Check sheet for the drawn part. Datum: minimum x, y, z corner. Units: mm. A direction names the side the tool comes from. Give positions to 0.01 mm unless a question says otherwise; leave off trailing zeros. Write each loop counter-clockwise with the first axis right and the second up, starting at its lowest first coordinate (ties: lowest second). Pieces come first, ordered by that corner, then holes. Notation, with made-up numbers: (42, 28.5) -> (85, 28.5) arc R12 cw to (85, 47.5) -> close; hole circle Ø7 at (64.25, -36). An arc over 180 degrees is marked (long way). Answer as CSV lines item,"result". Start each with the question number.
1) Gauge pin test, flat end, axial feed: pin 1 Ø5 at (x, y) = (59, 8) entering from +Z. Record the tip position at first contact, or that the pin passes through.
2) Sectioned sample at A-A on x = 10. Record the cut outline in (y, z), and give its area (3 significant figures).
3) Sectioned sample at B-B on y = 5.25. Record the cut outline in (x, z).
4) Tool access check on the marked faces 1 and 2. Record the directions out of +Z, -Z, +X, -X, +Y, -Y that give a thin tool (end or side, any length) a straight path to the whole face; none if there is none.
5) Mould release check, pull along X, two halves, no side actions. Record for the marked faces 3, 4 and 5: released by +X, released by -X, zero draft, split by the parting line, or undercut.
6) Material ranges on L1, parallel to Y at x = 61, z = 5.3; L2, parallel to Z at x = 11, y = 6.75; L3, parallel to X at y = 15.25, z = 4.5, recorded low to high.
7) Sectioned sample at C-C on x = 61. Record the cut outline in (y, z), and give its area (3 significant figures).
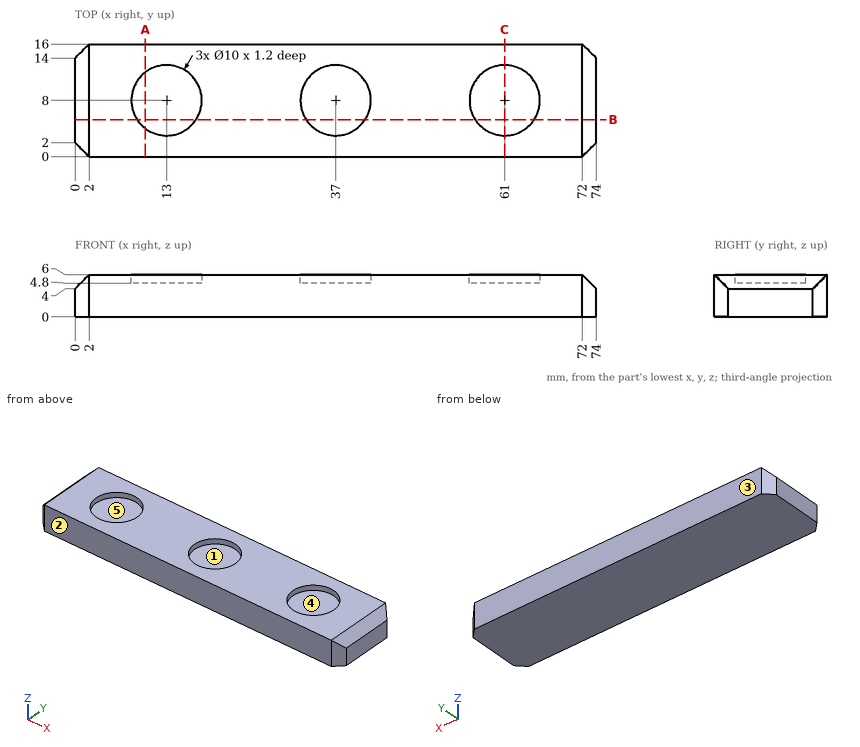
Ans:
1,pin 1,"stops at z = 4.8"
2,outline,"(0, 0) -> (16, 0) -> (16, 6) -> (12, 6) -> (12, 4.8) -> (4, 4.8) -> (4, 6) -> (0, 6) -> close"
2,area,"86.4 mm²"
3,outline,"(0, 0) -> (74, 0) -> (74, 4) -> (72, 6) -> (65.18, 6) -> (65.18, 4.8) -> (56.82, 4.8) -> (56.82, 6) -> (41.18, 6) -> (41.18, 4.8) -> (32.82, 4.8) -> (32.82, 6) -> (17.18, 6) -> (17.18, 4.8) -> (8.82, 4.8) -> (8.82, 6) -> (2, 6) -> (0, 4) -> close"
4,face 1,"+Z"
4,face 2,"+Z, -Z, +X, -X, -Y"
5,face 3,"zero draft"
5,face 4,"undercut"
5,face 5,"undercut"
6,L1,"y = 0 to 3, 13 to 16"
6,L2,"z = 0 to 4.8"
6,L3,"x = 1.25 to 72.75"
7,outline,"(0, 0) -> (16, 0) -> (16, 6) -> (13, 6) -> (13, 4.8) -> (3, 4.8) -> (3, 6) -> (0, 6) -> close"
7,area,"84.0 mm²"
